Design review of the part built by this model. Coordinates are the model's own, in mm. A direction names the side the tool comes from. Give positions to 0.01 mm unless a question says otherwise; leave off trailing zeros. Write each loop counter-clockwise with the first axis right and the second up, starting at its lowest first coordinate (ties: lowest second). Pieces come first, ordered by that corner, then holes. Notation, with made-up numbers: M 51.5,36.25 L 68.5,36.25 A8 cw 68.5,43.25 Z; hole C -36,-2.5 d10. An arc over 180 degrees is marked long. Use a Markdown table: item, result. Add a question column.
```python
from build123d import *

# Parameters (mm, degrees)
EXTRUDE_1_DEPTH     = 15
SKETCH_3_R          = 1.5
CUT_EXTRUDE_1_DEPTH = 23.216894472
RIB_1_REACH         = 36.185
SKETCH_4_WALL_W     = 83.349688256
SKETCH_4_WALL_H     = 3
SKETCH_5_R          = 1.5
CUT_EXTRUDE_2_DEPTH = 23.216894472
FILLET_1_R          = 3


with BuildPart() as part:
    # 草图2 → 拉伸-薄壁1 (new, symmetric)
    with BuildSketch(Plane.XY):
        Polygon((0, 14), (0, 0), (-8.52, 0), (-8.52, 2.5), (-2.5, 2.5), (-2.5, 14), align=None)
    extrude(amount=EXTRUDE_1_DEPTH, both=True)

    # 草图3 → 切除-拉伸1 (cut, through all)
    with BuildSketch(Plane.XZ):
        with Locations((-5.52, 0)):
            Circle(SKETCH_3_R)
    extrude(amount=-CUT_EXTRUDE_1_DEPTH, mode=Mode.SUBTRACT)

    # 草图4 wall → 筋1 (add, up to next)
    with BuildSketch(Plane(origin=(-5.51, 8.25, 15), x_dir=(-0.463776683525, -0.885952136302, 0), z_dir=(0.885952136302, -0.463776683525, 0)), mode=Mode.PRIVATE) as rib_1_sk1:
        with Locations((0, 1.5)):
            Rectangle(SKETCH_4_WALL_W, SKETCH_4_WALL_H)
    rib_1_tool1 = extrude(rib_1_sk1.sketch, amount=RIB_1_REACH, mode=Mode.PRIVATE) - part.part
    rib_1 = rib_1_tool1.solids().sort_by_distance((-5.51, 8.25, 15))[0]
    add(rib_1)

    # 镜向1: 筋1 across plane
    add(rib_1.mirror(Plane.XY))

    # 草图5 → 切除-拉伸2 (cut, through all)
    with BuildSketch(Plane(origin=(0, 0, 0), x_dir=(0, 0, -1), z_dir=(1, 0, 0))):
        with Locations((-9, 10)):
            Circle(SKETCH_5_R)
        with Locations((9, 10)):
            Circle(SKETCH_5_R)
    extrude(amount=-CUT_EXTRUDE_2_DEPTH, mode=Mode.SUBTRACT)

    # 圆角1
    fillet_1_edges = [part.edges().sort_by_distance(p)[0] for p in [
        (-5.51, 2.5, 12),
        (-5.51, 2.5, -12),
    ]]
    fillet(fillet_1_edges, radius=FILLET_1_R)


solid = part.part
```
(1) Machinability: for faces 1 (the flat face through (-5.47, 8.33, 13.29)), 2 (the flat face through (-6, 2.5, -2)), which of the approach directions +Z, -Z, +X, -X, +Y, -Y give a long, thin tool a straight path to every point of the face, cutting with its end or side? Answer none if there is none.
(2) For pin 1 (6 mm diameter, centred on y = 6, z = -3.5, fed in from -X), flat-tipped, find the tip position at first contact; note if it passes through.
(3) Add section B-B on y = 11. Give the boundary of the cut face in (x, z).
(4) The part is to be moulded in two halves that separate along X. For faces 3 (the flat face through (-3, 6, 15)), 4 (the flat face through (0, 7, 0)), 5 (the cylindrical face through (-6.71, 1.23, -0.91)), 6 (the flat face through (-8.52, 1, 0)), say which applies: released by +X, released by -X, zero draft, split by the parting line, or undercut.
(5) Add section C-C on x = -5.52. Give the boundary of the cut face in (y, z).
(6) Wall thickness on L1, parallel to Y at x = -0.75, z = 9; L2, parallel to Z at x = -5.52, y = 1.2; L3, parallel to Z at x = -2.75, y = 12.25: over which ranges is each line inside the solid? List them lowest first.
(7) Add section D-D on z = -0.75. Give the boundary of the cut face in (x, y), then the cut area to 3 significant figures.
(8) Add section A-A on x = -1.25. Give the boundary of the cut face in (y, z), then the cut area to 3 significant figures.
From the geometry:
| question | item | result |
|---|---|---|
| 1 | face 1 | +Z, -Z, -X, +Y |
| 1 | face 2 | -X, +Y |
| 2 | pin 1 | stops at x = -2.5 |
| 3 | outline | M -4.07,-15 L 0,-15 L 0,-10.12 L -2.5,-10.12 L -2.5,-12 L -4.07,-12 Z; M -4.07,12 L -2.5,12 L -2.5,10.12 L 0,10.12 L 0,15 L -4.07,15 Z; M -2.5,-7.88 L 0,-7.88 L 0,7.88 L -2.5,7.88 Z |
| 4 | face 3 | zero draft |
| 4 | face 4 | released by +X |
| 4 | face 5 | undercut |
| 4 | face 6 | released by -X |
| 5 | outline | M 0,-15 L 8.23,-15 L 8.23,-12 L 5.5,-12 A3 cw 2.5,-9 L 2.5,-1.5 L 0,-1.5 Z; M 0,1.5 L 2.5,1.5 L 2.5,9 A3 cw 5.5,12 L 8.23,12 L 8.23,15 L 0,15 Z |
| 6 | L1 | y = 0 to 8.5, 11.5 to 14 |
| 6 | L2 | z = -15 to -1.5, 1.5 to 15 |
| 6 | L3 | z = -15 to -12, 12 to 15 |
| 7 | outline | M -8.52,0 L -6.82,0 L -6.82,2.5 L -8.52,2.5 Z; M -4.22,0 L 0,0 L 0,14 L -2.5,14 L -2.5,2.5 L -4.22,2.5 Z |
| 7 | area | 43.6 mm^2 |
| 8 | outline | M 0,-15 L 14,-15 L 14,15 L 0,15 Z; hole C 10,-9 d3; hole C 10,9 d3 |
| 8 | area | 406 mm^2 |
